Geometry: final body of the model. Coordinates: model frame, mm. Give positions to 0.01 mm unless a question says otherwise; leave off trailing zeros. Use one line per item in the form item = value. Start each with the question number.
Item 1: Section query A-A on x = 50.8. Give the number of separate pieces and of enclosed holes in the cut face, then the cut area to 3 significant figures.
Item 2: Contact query for a flat-ended pin moving along its axis: P1, Ø6, axis at x = 25.4, z = 0, coming from the +Y side. Output: stop coordinate, or through.
Item 3: Material intervals for line 1 along Z through (x, y) = (0, 2.45); line 2 along X through (y, z) = (0.5, -24.5), sorted ascending. Write a range as from..to.
from build123d import *

# Parameters (mm, degrees)
SKETCH1_W                             = 127
SKETCH1_H                             = 127
BOSS_EXTRUDE1_DEPTH                   = 6.35
TAP_DRILL_FOR_1_4_20_TAP2_D           = 5.1054
TAP_DRILL_FOR_1_4_20_TAP2_CSINK_D     = 6.3754
TAP_DRILL_FOR_1_4_20_TAP2_CSINK_ANGLE = 90
LPATTERN1_COUNT                       = 5
LPATTERN1_PITCH                       = 25.4
LPATTERN1_COUNT_DIR2                  = 5
LPATTERN1_PITCH_DIR2                  = 25.4
CHAMFER1_SIZE                         = 7.62


with BuildPart() as part:
    # Sketch1 → Boss-Extrude1 (new body)
    with BuildSketch(Plane(origin=(0, 0, 0), x_dir=(1, 0, 0), z_dir=(0, 1, 0))):
        Rectangle(SKETCH1_W, SKETCH1_H)
    extrude(amount=BOSS_EXTRUDE1_DEPTH)

    # Tap Drill for 1/4-20 Tap2 (through all)
    with Locations(Plane(origin=(-50.8, 6.35, -50.8), x_dir=(0, 0, 1), z_dir=(0, 1, 0))):
        with Locations((0, 0)):
            tap_drill_for_1_4_20_tap2 = CounterSinkHole(TAP_DRILL_FOR_1_4_20_TAP2_D / 2, TAP_DRILL_FOR_1_4_20_TAP2_CSINK_D / 2, counter_sink_angle=TAP_DRILL_FOR_1_4_20_TAP2_CSINK_ANGLE)

    # LPattern1: Tap Drill for 1_4-20 Tap2 5 × 5
    with Locations(*[(j * LPATTERN1_PITCH_DIR2, 0, i * LPATTERN1_PITCH) for i in range(LPATTERN1_COUNT) for j in range(LPATTERN1_COUNT_DIR2) if (i, j) != (0, 0)]):
        add(tap_drill_for_1_4_20_tap2, mode=Mode.SUBTRACT)

    # Chamfer1
    chamfer1_edges = [part.edges().sort_by_distance(p)[0] for p in [
        (63.5, 3.175, 63.5),
        (-63.5, 3.175, 63.5),
        (-63.5, 3.175, -63.5),
        (63.5, 3.175, -63.5),
    ]]
    chamfer(chamfer1_edges, length=CHAMFER1_SIZE)


solid = part.part
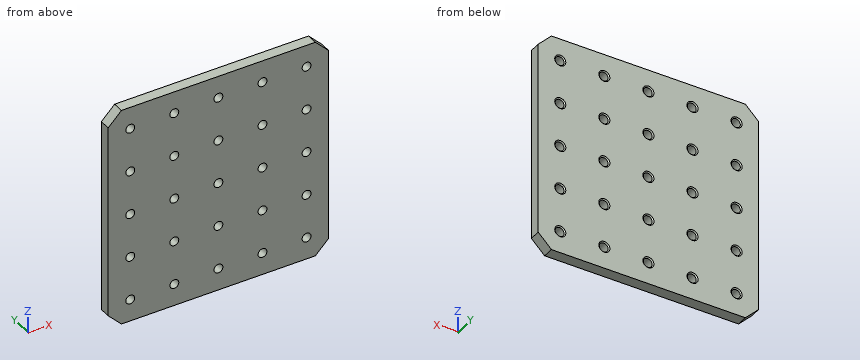
Answer sheet:
q1.separate_pieces = 6
q1.enclosed_holes = 0
q1.area = 642 mm2
q2.P1 = 6.16
q3.line_1 = -63.5..-53.35, -48.25..-27.95, -22.85..-2.55, 2.55..22.85, 27.95..48.25, 53.35..63.5
q3.line_2 = -63.5..-53.19, -48.41..-27.79, -23.01..-2.39, 2.39..23.01, 27.79..48.41, 53.19..63.5
